For this review, take the finished solid that the model builds, in its own axes (mm). Face numbers are marked on the shaded views. A direction names the side the tool comes from. Coordinates: 2 decimals unless noted, no trailing zeros. Write each loop counter-clockwise with the first axis right and the second up, starting at its lowest first coordinate (ties: lowest second). Pieces come first, ordered by that corner, then holes. Notation, with made-up numbers: (52, -3) -> (65, -3) arc R10 ccw to (65, 12) -> close; hole circle Ø1 at (50, -14). An arc over 180 degrees is marked (long way). One line per item, written item: value. Start each with the question number.
1) Add section B-B (x = -1.15). State the section outline as (y, z) points (3 decimals).
2) Add section C-C (y = -0.3). State how many separate pieces and enclosed holes the cut face has, and give its area (3 significant figures).
3) Add section A-A (z = 0.2). State the section outline as (x, y) points (3 decimals), and give its area (3 significant figures).
4) For pin 1 Ø0.5 at (y, z) = (-1.5, 0) entering from -X; pin 2 Ø1 at (x, z) = (0.5, -1) entering from -Y, all flat-tipped, find the tip position at first contact; note any pin that passes through.
5) Mouldability with a two-part tool opening along Z and no side actions: class the marked faces 5, 6 and 7 as released by +Z, released by -Z, zero draft, split by the parting line, or undercut.
6) Machinability: for the marked faces 1, 2, 3 and 4, which of the approach directions +Z, -Z, +X, -X, +Y, -Y give a long, thin tool a straight path to every point of the face, cutting with its end or side? Answer none if there is none.
7) For probe 1 along X at (y, z) = (0.8, 0); probe 2 along Z at (x, y) = (0, -0.4) (3 decimals); probe 3 along X at (y, z) = (-0.2, 0) (3 decimals), list the stretches that pass through material, from the lowest coordinate up. Write a range as from..to.
8) Add section D-D (x = 1.35). State the section outline as (y, z) points.
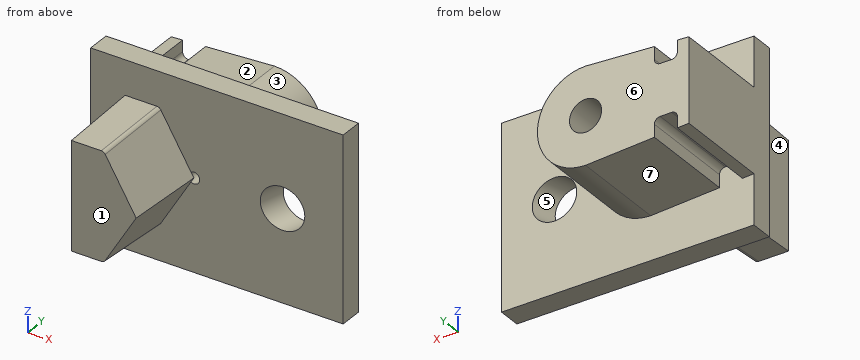
from build123d import *

# Parameters (mm, degrees)
BOSS_EXTRUDE1_DEPTH     = 2.125
SKETCH4_R               = 0.35
THROUGH_HOLES_DEPTH     = 4.445014514
FILLET1_R               = 0.125
SKETCH5_R               = 0.125
BOSS_EXTRUDE2_DEPTH     = 0.5
SKETCH8_R               = 0.46
CUT_EXTRUDE1_DEPTH      = 5.582575695
CUT_EXTRUDE2_DEPTH      = 5.367851302
CUT_EXTRUDE2_DEPTH_BACK = 5.367851302
SKETCH9_W               = 1.465031661
SKETCH9_H               = 4
BOSS_EXTRUDE3_DEPTH     = 1.75
CHAMFER1_SIZE           = 1.8
CHAMFER1_SIZE_2         = 0.078589697
FILLET2_R               = 0.1


with BuildPart() as part:
    # Sketch3 → Boss-Extrude1 (new body)
    with BuildSketch(Plane(origin=(0, 0, 0), x_dir=(1, 0, 0), z_dir=(0, 1, 0))):
        with BuildLine():
            Line((-2.5, 0.9), (-2, 0.93))
            Line((-2, 0.93), (-2, 0.56))
            Line((-2, 0.56), (-1.5, 0.56))
            Line((-1.5, 0.56), (-1.5, 0.96))
            Line((-1.5, 0.96), (0, 1.05))
            ThreePointArc((0, 1.05), (1.05, 0), (0, -1.05))
            Line((0, -1.05), (-1.5, -0.96))
            Line((-1.5, -0.96), (-1.5, -0.56))
            Line((-1.5, -0.56), (-2, -0.56))
            Line((-2, -0.56), (-2, -0.93))
            Line((-2, -0.93), (-2.5, -0.9))
            Line((-2.5, -0.9), (-2.5, 0.9))
        make_face()
    extrude(amount=BOSS_EXTRUDE1_DEPTH)

    # Sketch4 → Through Holes (cut, through all)
    with BuildSketch(Plane(origin=(0, 2.125, 0), x_dir=(1, 0, 0), z_dir=(0, 1, 0))):
        with Locations(Location((0, 0, 0), (0, 0, 270))):
            Circle(SKETCH4_R)
    extrude(amount=-THROUGH_HOLES_DEPTH, mode=Mode.SUBTRACT)

    # Fillet1
    fillet1_edges = [part.edges().sort_by_distance(p)[0] for p in [
        (-2, 1.0625, -0.56),
        (-1.5, 1.0625, -0.56),
        (-1.5, 1.0625, 0.56),
        (-2, 1.0625, 0.56),
    ]]
    fillet(fillet1_edges, radius=FILLET1_R)

    # Sketch5 → Boss-Extrude2 (add)
    with BuildSketch(Plane(origin=(0, 0, 0), x_dir=(1, 0, 0), z_dir=(0, 1, 0))):
        Polygon((-2.25, -2), (1.75, -2), (3.25, -2), (3.25, 2), (1.75, 2), (-2.25, 2), align=None)
        with Locations(Location((0, 0, 0), (0, 0, 270))):
            Circle(SKETCH5_R, mode=Mode.SUBTRACT)
    extrude(amount=-BOSS_EXTRUDE2_DEPTH)

    # Sketch8 → Cut-Extrude1 (cut, through all)
    with BuildSketch(Plane(origin=(0.7, 2.1, 0), x_dir=(0.948683298050514, -0.3162277660168378, 0), z_dir=(0.3162277660168378, 0.948683298050514, 0))):
        with Locations((1.987936011, 0)):
            Circle(SKETCH8_R)
    extrude(amount=-CUT_EXTRUDE1_DEPTH, mode=Mode.SUBTRACT)

    # Sketch9 → Cut-Extrude2 (cut, two sides: drawn at the far end of the back side and taken through both)
    with BuildSketch(Plane.XZ.offset(-CUT_EXTRUDE2_DEPTH_BACK)):
        with Locations((-2.982515831, 0)):
            Rectangle(SKETCH9_W, SKETCH9_H)
    extrude(amount=CUT_EXTRUDE2_DEPTH + CUT_EXTRUDE2_DEPTH_BACK, mode=Mode.SUBTRACT)

    # Sketch10 → Boss-Extrude3 (add)
    with BuildSketch(Plane.XZ.offset(0.5)):
        Polygon((-1.5, 1.25), (-1.5, -1.25), (-0.75, -1.25), (0, 0), (-0.75, 1.25), align=None)
    extrude(amount=BOSS_EXTRUDE3_DEPTH)

    # Chamfer1
    # the kernel refuses this chamfer: 1.8, 0.078589697 mm, written as the material it takes off along each edge
    with BuildSketch(Plane(origin=(-6.179835266, -2.25, -1.25), x_dir=(0, 0.999998592613724, -0.0016777278000430623), z_dir=(1, 0, 0))) as chamfer1_piece_1_section:
        Polygon((CHAMFER1_SIZE * 0.999998592614, CHAMFER1_SIZE * 0.00167772780004), (-CHAMFER1_SIZE_2 * 0.00167772780507, CHAMFER1_SIZE_2 * 0.999998595608), (0, 0), align=None)
    chamfer1_piece_1 = extrude(amount=10.109670532, mode=Mode.PRIVATE)
    chamfer1_piece_1 = split(chamfer1_piece_1, bisect_by=Plane(origin=(-1.125, -0.5, -1.243941513), z_dir=(0, -1, 0)), keep=Keep.TOP, mode=Mode.PRIVATE)
    add(chamfer1_piece_1, mode=Mode.SUBTRACT)
    with BuildSketch(Plane(origin=(-3.157755381, -2.25, -5.262925634), x_dir=(0.0014386397198082417, 0.9999985926137243, -0.0008631838318849449), z_dir=(0.5144957554275265, 0, 0.8574929257125442))) as chamfer1_piece_2_section:
        Polygon((CHAMFER1_SIZE * 0.999998592614, CHAMFER1_SIZE * 0.00167772780004), (-CHAMFER1_SIZE_2 * 0.00167772780507, CHAMFER1_SIZE_2 * 0.999998595608), (0, 0), align=None)
    chamfer1_piece_2 = extrude(amount=10.817408506, mode=Mode.PRIVATE)
    chamfer1_piece_2 = split(chamfer1_piece_2, bisect_by=Plane(origin=(-0.38019511, -0.5, -0.621882934), z_dir=(0, -1, 0)), keep=Keep.TOP, mode=Mode.PRIVATE)
    add(chamfer1_piece_2, mode=Mode.SUBTRACT)
    with BuildSketch(Plane(origin=(2.407755381, -2.25, -4.012925634), x_dir=(0.0014386397198082065, 0.9999985926137243, 0.0008631838318849242), z_dir=(-0.5144957554275267, 0, 0.8574929257125442))) as chamfer1_piece_3_section:
        Polygon((CHAMFER1_SIZE * 0.999998592614, CHAMFER1_SIZE * 0.00167772780004), (-CHAMFER1_SIZE_2 * 0.00167772780507, CHAMFER1_SIZE_2 * 0.999998595608), (0, 0), align=None)
    chamfer1_piece_3 = extrude(amount=10.817408506, mode=Mode.PRIVATE)
    chamfer1_piece_3 = split(chamfer1_piece_3, bisect_by=Plane(origin=(-0.38019511, -0.5, 0.621882934), z_dir=(0, -1, 0)), keep=Keep.TOP, mode=Mode.PRIVATE)
    add(chamfer1_piece_3, mode=Mode.SUBTRACT)
    with BuildSketch(Plane(origin=(3.929835266, -2.25, 1.25), x_dir=(0, 0.999998592613724, 0.0016777278000430623), z_dir=(-1, 0, 0))) as chamfer1_piece_4_section:
        Polygon((CHAMFER1_SIZE * 0.999998592614, CHAMFER1_SIZE * 0.00167772780004), (-CHAMFER1_SIZE_2 * 0.00167772780507, CHAMFER1_SIZE_2 * 0.999998595608), (0, 0), align=None)
    chamfer1_piece_4 = extrude(amount=10.109670532, mode=Mode.PRIVATE)
    chamfer1_piece_4 = split(chamfer1_piece_4, bisect_by=Plane(origin=(-1.125, -0.5, 1.243941513), z_dir=(0, -1, 0)), keep=Keep.TOP, mode=Mode.PRIVATE)
    add(chamfer1_piece_4, mode=Mode.SUBTRACT)

    # Fillet2
    fillet2_edges = [part.edges().sort_by_distance(p)[0] for p in [
        (-0.772866375, -1.375, 1.209613628),
        (-0.772866375, -1.375, -1.209613628),
    ]]
    fillet(fillet2_edges, radius=FILLET2_R)


solid = part.part
Numbers:
1. outline: (-2.25, -1.171) -> (-0.5, -1.248) -> (-0.5, -2) -> (0, -2) -> (0, -0.981) -> (2.125, -0.981) -> (2.125, 0.981) -> (0, 0.981) -> (0, 2) -> (-0.5, 2) -> (-0.5, 1.248) -> (-2.25, 1.171) -> close
2. separate pieces: 1
2. enclosed holes: 2
2. area: 21.3 mm²
3. outline: (-2.25, -0.5) -> (-1.5, -0.5) -> (-1.5, -2.25) -> (-0.212, -2.25) -> (-0.123, -0.5) -> (1.492, -0.5) -> (1.659, 0) -> (1.031, 0) -> (1.031, 2.125) -> (0.287, 2.125) -> (0.287, 0) -> (-0.287, 0) -> (-0.287, 2.125) -> (-2.25, 2.125) -> close; (2.365, -0.5) -> (3.25, -0.5) -> (3.25, 0) -> (2.532, 0) -> close
3. area: 10.4 mm²
4. pin 1: x = -1.5
4. pin 2: y = -0.5
5. face 5: undercut
5. face 6: zero draft
5. face 7: released by -Z
6. face 1: +Z, -Z, +X, -X, -Y
6. face 2: +Z, -X, +Y
6. face 3: +X, +Y
6. face 4: +Z, -Z, -X, -Y
7. probe 1: -2.25..-0.35, 0.35..1.05
7. probe 2: -2..-0.125, 0.125..2
7. probe 3: -2.25..-0.125, 0.125..1.544, 2.514..3.25
8. outline: (-0.5, -2) -> (0, -2) -> (0, 2) -> (-0.5, 2) -> close
